```python
from build123d import *


with BuildPart() as part:
    # AdditivePipe: sweep along a path in Sketch001
    with BuildLine(Plane.XY) as additivepipe_path:
        Line((0, 0), (-12.3, 0))
        ThreePointArc((-12.3, 0), (-14.42132, -0.87868), (-15.3, -3))
        Line((-15.3, -3), (-15.3, -73.5))
    # Sketch → AdditivePipe (sweep)
    with BuildSketch(Plane.YZ):
        Polygon((0, 0.733235), (-0.635, 0.366617), (-0.635, -0.366617), (0, -0.733235), (0.635, -0.366617), (0.635, 0.366617), align=None)
    sweep(path=additivepipe_path.line)


solid = part.part
```
Verification items for the finished model (mm, model axes). Give positions to 0.01 mm unless a question says otherwise; leave off trailing zeros. Loops run counter-clockwise (first coordinate to the right, second up) from the corner with the lowest first, then second, coordinate; pieces in that order, holes last.
1. Go/stop test with flat-tipped pins: pin 1 Ø0.6 at (y, z) = (-30, 0) entering from +X (3 decimals); pin 2 Ø0.6 at (x, z) = (-6, 0) entering from -Y (3 decimals). Record where each tip stops, or that it passes through.
2. Section check B-B, the plane x = -10. Enter the section's corners in (y, z) (3 decimals).
3. Section check C-C, the plane y = -9. Enter the section's corners in (x, z) (3 decimals).
4. Section check A-A, the plane z = 0.1. Enter the section's corners in (x, y) (3 decimals).
5. Thickness scan on line 1 (X direction, y = -8, z = 0.1) (3 decimals); line 2 (Y direction, x = -10.5, z = 0.3) (3 decimals); line 3 (X direction, y = -49, z = 0.65). Record the ranges inside material, lowest first.
Geometry says:
1. pin 1: stops at x = -14.665
1. pin 2: stops at y = -0.635
2. outline: (-0.635, -0.367) - (0, -0.733) - (0.635, -0.367) - (0.635, 0.367) - (0, 0.733) - (-0.635, 0.367) - close
3. outline: (-15.935, -0.367) - (-15.3, -0.733) - (-14.665, -0.367) - (-14.665, 0.367) - (-15.3, 0.733) - (-15.935, 0.367) - close
4. outline: (-15.935, -73.5) - (-14.665, -73.5) - (-14.665, -3) arc R2.365 cw to (-12.3, -0.635) - (0, -0.635) - (0, 0.635) - (-12.3, 0.635) arc R3.635 ccw to (-15.935, -3) - close
5. line 1: x = -15.935 to -14.665
5. line 2: y = -0.635 to 0.635
5. line 3: x = -15.44 to -15.16
